```python
from build123d import *

# Parameters (mm, degrees)
SKETCH1_R           = 4
EXTRUDE1_DEPTH      = 10
SKETCH2_R           = 7
EXTRUDE2_DEPTH      = 3
CHAMFER1_SIZE       = 0.6
SKETCH3_R           = 1
EXTRUDE3_DEPTH      = 8
EXTRUDE3_DEPTH_BACK = 8
CHAMFER2_SIZE       = 0.4


with BuildPart() as part:
    # Sketch1 → Extrude1 (new body, symmetric)
    with BuildSketch(Plane.XY):
        Circle(SKETCH1_R)
    extrude(amount=EXTRUDE1_DEPTH, both=True)

    # Sketch2 → Extrude2 (add)
    with BuildSketch(Plane.XY.offset(10)):
        Circle(SKETCH2_R)
    extrude(amount=EXTRUDE2_DEPTH)

    # Chamfer1
    chamfer1_edges = [part.edges().sort_by_distance(p)[0] for p in [
        (-7, 0, 13),
    ]]
    chamfer(chamfer1_edges, length=CHAMFER1_SIZE)

    # Sketch3 → Extrude3 (cut, two sides)
    with BuildSketch(Plane(origin=(0, 0, 0), x_dir=(0, 0, -1), z_dir=(1, 0, 0))) as extrude3_sk:
        with Locations((6, 0)):
            Circle(SKETCH3_R)
    extrude(amount=EXTRUDE3_DEPTH, mode=Mode.SUBTRACT)
    extrude(extrude3_sk.sketch, amount=-EXTRUDE3_DEPTH_BACK, mode=Mode.SUBTRACT)

    # Chamfer2
    chamfer2_edges = [part.edges().sort_by_distance(p)[0] for p in [
        (-4, 0, -10),
    ]]
    chamfer(chamfer2_edges, length=CHAMFER2_SIZE)


solid = part.part
```
Verification items for the finished model (mm, model axes). A direction names the side the tool comes from. Give positions to 0.01 mm unless a question says otherwise; leave off trailing zeros. Loops run counter-clockwise (first coordinate to the right, second up) from the corner with the lowest first, then second, coordinate; pieces in that order, holes last. Notation, with made-up numbers: M 78,27 L 101,27 A25 cw 101,51 Z; hole C 39.5,-19.75 d2. An arc over 180 degrees is marked long. Return JSON: item names as keys, results as strings.
1) Section check B-B, the plane z = 8.75. Enter the section's corners in (x, y), and give its area (3 significant figures).
Findings:
{"outline": "C 0,0 d8", "area": "50.3 mm2"}
2) Material ranges on L1, parallel to Z at x = -4.5, y = -0.25; L2, parallel to Y at x = -0.8, z = -6; L3, parallel to Y at x = -2.5, z = -6, recorded low to high. Write a range as [from, to].
Findings:
{"L1": "z = [10, 13]", "L2": "y = [-3.92, -1], [1, 3.92]", "L3": "y = [-3.12, -1], [1, 3.12]"}
3) Gauge pin test, flat ends, axial feed: P1, Ø1.5, axis at y = -3, z = 4.5, coming from the +X side; P2, Ø3, axis at y = 0, z = -6, coming from the -X side; P3, Ø6, axis at x = -1.5, z = 5, coming from the -Y side. Record the tip position at first contact, or that the pin passes through.
Findings:
{"P1": "stops at x = 3.31", "P2": "stops at x = -4", "P3": "stops at y = -4"}
4) Section check C-C, the plane z = -6. Enter the section's corners in (x, y), and give its area (3 significant figures).
Findings:
{"outline": "M -3.87,-1 A4 ccw 3.87,-1 Z; M -3.87,1 L 3.87,1 A4 ccw Z", "area": "34.4 mm2"}
5) Section check A-A, the plane y = 0. Enter the section's corners in (x, z).
Findings:
{"outline": "M -7,10 L -4,10 L -4,-5 L 4,-5 L 4,10 L 7,10 L 7,12.4 L 6.4,13 L -6.4,13 L -7,12.4 Z; M -4,-9.6 L -3.6,-10 L 3.6,-10 L 4,-9.6 L 4,-7 L -4,-7 Z"}
6) Tool access check on faces 1 (the flat face through (3, -3, 10)), 2 (the flat face through (0, 0, -10)). Record the directions out of +Z, -Z, +X, -X, +Y, -Y that give a thin tool (end or side, any length) a straight path to the whole face; none if there is none.
Findings:
{"face 1": "-Z", "face 2": "-Z, +X, -X, +Y, -Y"}
